Build history of the part. All positions in model axes, mm. Face numbers are marked on the shaded views. A direction names the side the tool comes from. Round coordinates to 2 decimals unless told otherwise and drop trailing zeros. Loops run counter-clockwise (first coordinate to the right, second up) from the corner with the lowest first, then second, coordinate; pieces in that order, holes last.
from build123d import *

# Parameters (mm, degrees)
F0_W     = 2
F0_H     = 10
F1_DEPTH = 2.3368
F2_DEPTH = 2.0066
F4_DEPTH = 2
F6_DEPTH = 7
F8_D     = 1


# Not quite as in the source:
# - a feature names something its author has since deleted; it is built from what else it names


with BuildPart() as f1:
    # F0 (on Top) → F1 (new body)
    with BuildSketch(Plane.XY):
        with Locations((-18.8875418854, 5)):
            Rectangle(F0_W, F0_H)
        with Locations((-8.8875418854, 5)):
            Rectangle(F0_W, F0_H)
        Polygon((-17.8550429996, 21.3176092022), (-15.8875418854, 20.9585279226), (-15.8875418854, 22.9585279226), align=None)
        Polygon((-11.8875418854, 22.9585279226), (-11.8875418854, 20.9585279226), (-9.9200407711, 21.3176092022), align=None)
        Polygon((-11.8875418854, 20.9585279226), (-9.8875418854, 10), (-7.8875418854, 10), (-9.9200407711, 21.3176092022), align=None)
        Polygon((-15.8875418854, 20.9585279226), (-13.8875418854, 20.9585279226), (-11.8875418854, 20.9585279226), (-11.8875418854, 22.9585279226), (-15.8875418854, 22.9585279226), align=None)
        Polygon((-19.8875418854, 10), (-17.8875418854, 10), (-15.8875418854, 20.9585279226), (-17.8550429996, 21.3176092022), align=None)
    extrude(amount=-F1_DEPTH)

    # F0 (on Top) → F2 (join)
    with BuildSketch(Plane.XY):
        Polygon((-17.8875418854, 10), (-17.8875418854, 0), (-13.8875418854, 0), (-13.8875418854, 20.9585279226), (-15.8875418854, 20.9585279226), align=None)
        with Locations((-18.8875418854, 5)):
            Rectangle(F0_W, F0_H)
        Polygon((-13.8875418854, 20.9585279226), (-13.8875418854, 0), (-9.8875418854, 0), (-9.8875418854, 10), (-11.8875418854, 20.9585279226), align=None)
        Polygon((-19.8875418854, 10), (-17.8875418854, 10), (-15.8875418854, 20.9585279226), (-17.8550429996, 21.3176092022), align=None)
        with Locations((-8.8875418854, 5)):
            Rectangle(F0_W, F0_H)
        Polygon((-15.8875418854, 20.9585279226), (-13.8875418854, 20.9585279226), (-11.8875418854, 20.9585279226), (-11.8875418854, 22.9585279226), (-15.8875418854, 22.9585279226), align=None)
        Polygon((-17.8550429996, 21.3176092022), (-15.8875418854, 20.9585279226), (-15.8875418854, 22.9585279226), align=None)
        Polygon((-11.8875418854, 20.9585279226), (-9.8875418854, 10), (-7.8875418854, 10), (-9.9200407711, 21.3176092022), align=None)
        Polygon((-11.8875418854, 22.9585279226), (-11.8875418854, 20.9585279226), (-9.9200407711, 21.3176092022), align=None)
    extrude(amount=F2_DEPTH)

    # F3 (on face) → F4 (join)
    with BuildSketch(Plane(origin=(0, 0, -2.3368), x_dir=(1, 0, 0), z_dir=(0, 0, -1))):
        Polygon((-14.3875418854, 0), (-17.8875418854, 0), (-17.8875418854, -10), (-15.8875418854, -20.9585279226), (-11.8875418854, -20.9585279226), (-9.8875418854, -10), (-9.8875418854, 0), align=None)
        with BuildLine():
            ThreePointArc((-13.8875418854, -11), (-14.7410952759, -11.3535533906), (-14.3875418854, -10.5))
            ThreePointArc((-14.3875418854, -10.5), (-14.0339884948, -10.6464466094), (-13.8875418854, -11))
        make_face(mode=Mode.SUBTRACT)
        with BuildLine():
            ThreePointArc((-14.3875418854, -2.5), (-14.8875418854, -2), (-14.3875418854, -1.5))
            ThreePointArc((-14.3875418854, -1.5), (-14.0339884948, -1.6464466094), (-13.8875418854, -2))
            ThreePointArc((-13.8875418854, -2), (-14.0339884948, -2.3535533906), (-14.3875418854, -2.5))
        make_face(mode=Mode.SUBTRACT)
        Polygon((-17.8875418854, 0), (-19.8875418854, 0), (-19.8875418854, -10), (-17.8550429996, -21.3176092022), (-15.8875418854, -22.9585279226), (-11.8875418854, -22.9585279226), (-9.9200407711, -21.3176092022), (-7.8875418854, -10), (-7.8875418854, 0), (-9.8875418854, 0), (-9.8875418854, -10), (-11.8875418854, -20.9585279226), (-15.8875418854, -20.9585279226), (-17.8875418854, -10), align=None)
    extrude(amount=F4_DEPTH)

    # F5 (on face) → F6 (join)
    with BuildSketch(Plane.XY.offset(2.0066)):
        Polygon((-13.3875418854, 22.9585279226), (-13.3875418854, 0), (-11.3875418854, 0), (-11.3875418854, 22.5415221307), (-11.8875418854, 22.9585279226), align=None)
        Polygon((-16.3875418854, 0), (-14.3875418854, 0), (-14.3875418854, 22.9585279226), (-15.8875418854, 22.9585279226), (-16.3875418854, 22.5415221307), align=None)
    extrude(amount=F6_DEPTH)

    # F8 (through all)
    with Locations(Plane.YZ.offset(-11.3875418854)):
        with Locations((3, 5.5066), (19.5415221307, 5.5066)):
            Hole(F8_D / 2)


solid = f1.part
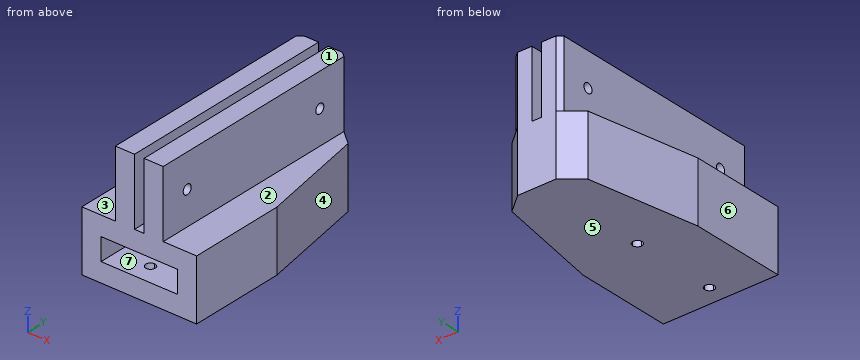
(1) Slice it at D-D on y = 5.5. List the corners of the cut face in (x, z).
Responses:
outline: (-19.89, -4.34) - (-7.89, -4.34) - (-7.89, 2.01) - (-11.39, 2.01) - (-11.39, 9.01) - (-13.39, 9.01) - (-13.39, 2.01) - (-14.39, 2.01) - (-14.39, 9.01) - (-16.39, 9.01) - (-16.39, 2.01) - (-19.89, 2.01) - close; hole (-17.89, -2.34) - (-9.89, -2.34) - (-9.89, 0) - (-17.89, 0) - close
(2) Slice it at B-B on z = 7.5. List the corners of the cut face in (x, y).
Responses:
outline: (-16.39, 0) - (-14.39, 0) - (-14.39, 22.96) - (-15.89, 22.96) - (-16.39, 22.54) - close; (-13.39, 0) - (-11.39, 0) - (-11.39, 22.54) - (-11.89, 22.96) - (-13.39, 22.96) - close
(3) Probe line 1 (Z direction, x = -11.9, y = 3); line 2 (Z direction, x = -16.25, y = 18.5); line 3 (X direction, y = 9.25, z = -1). List the from-to ranges inside material, lowest first.
Responses:
line 1: z = -4.34 to -2.34, 0 to 5.01, 6.01 to 9.01
line 2: z = -4.34 to -2.34, 0 to 9.01
line 3: x = -19.89 to -17.89, -9.89 to -7.89
(4) Slice it at A-A on y = 3. List the corners of the cut face in (x, z), plus the area to 3 significant figures.
Responses:
outline: (-19.89, -4.34) - (-7.89, -4.34) - (-7.89, 2.01) - (-11.39, 2.01) - (-11.39, 5.01) - (-13.39, 5.01) - (-13.39, 2.01) - (-14.39, 2.01) - (-14.39, 5.01) - (-16.39, 5.01) - (-16.39, 2.01) - (-19.89, 2.01) - close; (-16.39, 6.01) - (-14.39, 6.01) - (-14.39, 9.01) - (-16.39, 9.01) - close; (-13.39, 6.01) - (-11.39, 6.01) - (-11.39, 9.01) - (-13.39, 9.01) - close; hole (-17.89, -2.34) - (-9.89, -2.34) - (-9.89, 0) - (-17.89, 0) - close
area: 81.4 mm2
(5) Which spindle directions (+Z, -Z, +X, -X, +Y, -Y) get a long thin tool onto all of the face, cutting with end or side? Do the marked faces 1, 2 and 3. Say none if no direction does.
Responses:
face 1: +Z, +X, -X, +Y, -Y
face 2: +Z, +X, +Y, -Y
face 3: +Z, -X, +Y, -Y
(6) Pin check, flat tips, straight feed: P1, Ø6, axis at x = -14, z = -1, coming from the -Y side; P2, Ø7.5, axis at y = 7, z = 6.5, coming from the -X side; P3, Ø3.5, axis at y = 16, z = 6.5, coming from the +X side; P4, Ø8, axis at y = 17, z = -0.5, coming from the -X side. Stop position of each tip, or through.
Responses:
P1: stops at y = 0
P2: stops at x = -16.39
P3: stops at x = -11.39
P4: stops at x = -19.35
(7) Slice it at C-C on x = -13. List the corners of the cut face in (y, z).
Responses:
outline: (0, -4.34) - (22.96, -4.34) - (22.96, 9.01) - (0, 9.01) - (0, 0) - (20.96, 0) - (20.96, -2.34) - (0, -2.34) - close; hole circle Ø1 at (3, 5.51); hole circle Ø1 at (19.54, 5.51)
(8) Pull direction X, two halves, no side cores. Call the marked faces 4, 5, 6 and 7: +X half, -X half, draft (parallel to the pull), parting line (faces both ways), or undercut.
Responses:
face 4: +X half
face 5: draft
face 6: -X half
face 7: undercut
